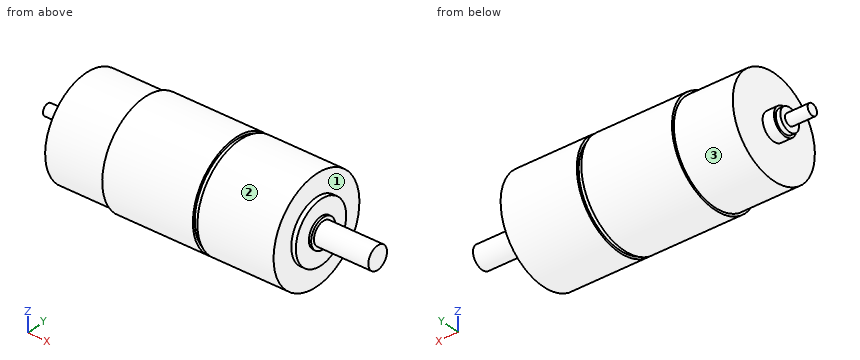
from build123d import *


with BuildPart() as part:
    # Sketch1 → Revolve1 (revolve)
    with BuildSketch(Plane(origin=(0, 0, 0), x_dir=(1, 0, 0), z_dir=(0, 1, 0)), mode=Mode.PRIVATE) as revolve1_sk:
        Polygon((0, 2.5), (0, 0), (19, 0), (19, 20), (116.6, 20), (116.6, 0), (145.6, 0), (145.6, 5), (121.6, 5), (121.6, 6.5), (120.6, 6.5), (120.6, 13.5), (118.6, 13.5), (118.6, 23), (85, 23), (85, 22), (83, 22), (83, 23), (43, 23), (43, 22), (19, 22), (17, 22), (17, 6), (12, 6), (12, 5), (10, 5), (10, 2.5), align=None)
    revolve(revolve1_sk.sketch.rotate(Axis((0, 0, 0), (1, 0, 0)), 180), axis=Axis((0, 0, 0), (1, 0, 0)))


solid = part.part
Geometry: final body of the model. Coordinates: model frame, mm. Face numbers are marked on the shaded views. A direction names the side the tool comes from. Give positions to 0.01 mm unless a question says otherwise; leave off trailing zeros. Order: outer loops, then holes, each group sorted by start corner. A loop starts at its lowest first (then second) coordinate and runs counter-clockwise, first axis right, second up. Notation, with made-up numbers: (80, 56.25) -> (134, 56.25) arc R15 cw to (134, 76.25) -> close; hole circle Ø2 at (41.5, -32.75). An arc over 180 degrees is marked (long way). Put each result on its own line as item: value.
Q1. Material intervals for L1, parallel to Y at x = 90, z = 0; L2, parallel to X at y = -18.5, z = -4; L3, parallel to X at y = 1.5, z = 0.5, sorted ascending.
Here are the results:
L1: y = -23 to -20, 20 to 23
L2: x = 17 to 19, 116.6 to 118.6
L3: x = 0 to 19, 116.6 to 145.6
Q2. Reachability of the marked faces 1, 2 and 3 from +Z, -Z, +X, -X, +Y, -Y: full face, straight path, thin tool, end or side. Return the list, or none.
Here are the results:
face 1: +X
face 2: +X, -X
face 3: -X
Q3. Section D-D, the plane y = -11. Return loops of the section in (x, z).
Here are the results:
outline: (17, -19.05) -> (43, -19.05) -> (43, -20.2) -> (83, -20.2) -> (83, -19.05) -> (85, -19.05) -> (85, -20.2) -> (118.6, -20.2) -> (118.6, -7.83) -> (120.6, -7.83) -> (120.6, 7.83) -> (118.6, 7.83) -> (118.6, 20.2) -> (85, 20.2) -> (85, 19.05) -> (83, 19.05) -> (83, 20.2) -> (43, 20.2) -> (43, 19.05) -> (17, 19.05) -> close; hole (19, -16.7) -> (116.6, -16.7) -> (116.6, 16.7) -> (19, 16.7) -> close
Q4. Section C-C, the plane x = 96.5. Return loops of the section in (y, z), then the cut area to 3 significant figures.
Here are the results:
outline: circle Ø46 at (0, 0); hole circle Ø40 at (0, 0)
area: 405 mm^2
Q5. Pin query (flat end, axial travel): pin 1 (6 mm diameter, centred on x = 36, y = 14.5, fed in from -Z) (3 decimals); pin 2 (3 mm diameter, centred on x = 27, y = -9, fed in from +Z); pin 3 (12 mm diameter, centred on y = 11, z = -14.5, fed in from -X). Return the tip coordinate at first contact, or that it passes through.
Here are the results:
pin 1: stops at z = -18.755
pin 2: stops at z = 20.68
pin 3: stops at x = 17
Q6. Section A-A, the plane z = -15. Return loops of the section in (x, y), then the cut area to 4 significant figures.
Here are the results:
outline: (17, -16.09) -> (43, -16.09) -> (43, -17.44) -> (83, -17.44) -> (83, -16.09) -> (85, -16.09) -> (85, -17.44) -> (118.6, -17.44) -> (118.6, 17.44) -> (85, 17.44) -> (85, 16.09) -> (83, 16.09) -> (83, 17.44) -> (43, 17.44) -> (43, 16.09) -> (17, 16.09) -> close; hole (19, -13.23) -> (116.6, -13.23) -> (116.6, 13.23) -> (19, 13.23) -> close
area: 885.5 mm^2
Q7. Section B-B, the plane y = 10. Return loops of the section in (x, z), then the cut area to 3 significant figures.
Here are the results:
outline: (17, -19.6) -> (43, -19.6) -> (43, -20.71) -> (83, -20.71) -> (83, -19.6) -> (85, -19.6) -> (85, -20.71) -> (118.6, -20.71) -> (118.6, -9.07) -> (120.6, -9.07) -> (120.6, 9.07) -> (118.6, 9.07) -> (118.6, 20.71) -> (85, 20.71) -> (85, 19.6) -> (83, 19.6) -> (83, 20.71) -> (43, 20.71) -> (43, 19.6) -> (17, 19.6) -> close; hole (19, -17.32) -> (116.6, -17.32) -> (116.6, 17.32) -> (19, 17.32) -> close
area: 802 mm^2
